from build123d import *

# Parameters (mm, degrees)
SKETCH1_W           = 85
SKETCH1_H           = 77
BOSS_EXTRUDE1_DEPTH = 1.75
SKETCH3_R           = 17.907
SKETCH3_R_2         = 13.97
BOSS_EXTRUDE3_DEPTH = 4.7625
BOSS_EXTRUDE7_DEPTH = 26
SKETCH6_W           = 77
SKETCH6_H           = 5
BOSS_EXTRUDE8_DEPTH = 2.5


with BuildPart() as part:
    # Sketch1 → Boss-Extrude1 (new body)
    with BuildSketch(Plane(origin=(0, 0, 0), x_dir=(1, 0, 0), z_dir=(0, 1, 0))):
        Rectangle(SKETCH1_W, SKETCH1_H)
    extrude(amount=BOSS_EXTRUDE1_DEPTH)

    # Sketch3 → Boss-Extrude3 (add)
    with BuildSketch(Plane(origin=(0, 1.75, 0), x_dir=(1, 0, 0), z_dir=(0, 1, 0))):
        with Locations((19.133331774, 19.92813227)):
            Circle(SKETCH3_R)
        with Locations((19.133331774, 19.92813227)):
            Circle(SKETCH3_R_2, mode=Mode.SUBTRACT)
        with Locations((-19.133331774, 19.92813227)):
            Circle(SKETCH3_R)
        with Locations((-19.133331774, 19.92813227)):
            Circle(SKETCH3_R_2, mode=Mode.SUBTRACT)
    extrude(amount=BOSS_EXTRUDE3_DEPTH)

    # Sketch4 → Boss-Extrude7 (add)
    with BuildSketch(Plane(origin=(0, 1.75, 0), x_dir=(1, 0, 0), z_dir=(0, 1, 0))):
        with BuildLine():
            ThreePointArc((-34.668002675, 28.83513227), (-31.887785522, 32.497323119), (-28.266663548, 35.330823584))
            Line((-28.266663548, 35.330823584), (-28.266663548, 37.83513227))
            Line((-28.266663548, 37.83513227), (-38.266663548, 37.83513227))
            Line((-38.266663548, 37.83513227), (-38.266663548, 28.83513227))
            Line((-38.266663548, 28.83513227), (-34.668002675, 28.83513227))
        make_face()
        with BuildLine():
            ThreePointArc((-28.266663548, 4.525440956), (-31.887785522, 7.358941421), (-34.668002675, 11.02113227))
            Line((-34.668002675, 11.02113227), (-38.266663548, 11.02113227))
            Line((-38.266663548, 11.02113227), (-38.266663548, 2.02113227))
            Line((-38.266663548, 2.02113227), (-28.266663548, 2.02113227))
            Line((-28.266663548, 2.02113227), (-28.266663548, 4.525440956))
        make_face()
        with BuildLine():
            Line((0, 11.02113227), (-3.598660873, 11.02113227))
            ThreePointArc((-3.598660873, 11.02113227), (-6.378878026, 7.358941421), (-10, 4.525440956))
            Line((-10, 4.525440956), (-10, 2.02113227))
            Line((-10, 2.02113227), (0, 2.02113227))
            Line((0, 2.02113227), (0, 11.02113227))
        make_face()
        with BuildLine():
            ThreePointArc((10, 4.525440956), (6.378878026, 7.358941421), (3.598660873, 11.02113227))
            Line((3.598660873, 11.02113227), (0, 11.02113227))
            Line((0, 11.02113227), (0, 2.02113227))
            Line((0, 2.02113227), (10, 2.02113227))
            Line((10, 2.02113227), (10, 4.525440956))
        make_face()
        with BuildLine():
            Line((0, 28.83513227), (0, 37.83513227))
            Line((0, 37.83513227), (-10, 37.83513227))
            Line((-10, 37.83513227), (-10, 35.330823584))
            ThreePointArc((-10, 35.330823584), (-6.378878026, 32.497323119), (-3.598660873, 28.83513227))
            Line((-3.598660873, 28.83513227), (0, 28.83513227))
        make_face()
        with BuildLine():
            Line((10, 37.83513227), (0, 37.83513227))
            Line((0, 37.83513227), (0, 28.83513227))
            Line((0, 28.83513227), (3.598660873, 28.83513227))
            ThreePointArc((3.598660873, 28.83513227), (6.378878026, 32.497323119), (10, 35.330823584))
            Line((10, 35.330823584), (10, 37.83513227))
        make_face()
        with BuildLine():
            Line((28.266663548, 37.83513227), (28.266663548, 35.330823584))
            ThreePointArc((28.266663548, 35.330823584), (31.887785522, 32.497323119), (34.668002675, 28.83513227))
            Line((34.668002675, 28.83513227), (38.266663548, 28.83513227))
            Line((38.266663548, 28.83513227), (38.266663548, 37.83513227))
            Line((38.266663548, 37.83513227), (28.266663548, 37.83513227))
        make_face()
        with BuildLine():
            ThreePointArc((34.668002675, 11.02113227), (31.887785522, 7.358941421), (28.266663548, 4.525440956))
            Line((28.266663548, 4.525440956), (28.266663548, 2.02113227))
            Line((28.266663548, 2.02113227), (38.266663548, 2.02113227))
            Line((38.266663548, 2.02113227), (38.266663548, 11.02113227))
            Line((38.266663548, 11.02113227), (34.668002675, 11.02113227))
        make_face()
    extrude(amount=BOSS_EXTRUDE7_DEPTH)

    # Sketch6 → Boss-Extrude8 (add)
    with BuildSketch(Plane.ZY.offset(42.5)):
        with Locations((0, -0.75)):
            Rectangle(SKETCH6_W, SKETCH6_H)
    boss_extrude8 = extrude(amount=BOSS_EXTRUDE8_DEPTH)

    # Mirror1: Boss-Extrude8 across plane
    add(boss_extrude8.mirror(Plane(origin=(0, 0, 0), x_dir=(0, 0, 1), z_dir=(1, 0, 0))))


solid = part.part
Geometry check sheet. Reference: the model listing, model coordinates, mm. A direction names the side the tool comes from. Round coordinates to 2 decimals unless told otherwise and drop trailing zeros. Order: outer loops, then holes, each group sorted by start corner. A loop starts at its lowest first (then second) coordinate and runs counter-clockwise, first axis right, second up. Notation, with made-up numbers: (-36, 39.5) -> (-15, 39.5) arc R35 cw to (-15, 74.5) -> close; hole circle Ø10 at (-29, 46.25). An arc over 180 degrees is marked (long way). Use one line per item in the form item = value.
1. Go/stop test with flat-tipped pins: pin 1 (6 mm diameter, centred on x = 1.5, z = -16, fed in from +Y); pin 2 (1 mm diameter, centred on x = 8, z = 23, fed in from -Y); pin 3 (3 mm diameter, centred on y = 16, z = -36.5, fed in from -X); pin 4 (2 mm diameter, centred on x = 34, z = -10.5, fed in from +Y). Record where each tip stops, or that it passes through.
Working result:
pin_1 = 6.51
pin_2 = 0
pin_3 = -38.27
pin_4 = 27.75
2. Set-up check for faces 4 (the face through (-38.267, 15, -7)), 5 (the face through (44, -3.25, -1)), 6 (the face through (31.842, 16.983, -32.543)): record each of +Z, -Z, +X, -X, +Y, -Y from which the full face is reachable in a straight line by a thin tool's end or side.
Working result:
face_4 = +Z, -Z, -X, +Y
face_5 = +Z, -Z, +X, -X, -Y
face_6 = +Y
3. Scan lines: line 1 along Z through (x, y) = (3, 22); line 2 along X through (y, z) = (-1.5, 11.5); line 3 along X through (y, z) = (24.5, -29). Record each from-to range of solid material in increasing order. Write a range as from..to.
Working result:
line_1 = -37.84..-28.84, -11.02..-2.02
line_2 = -45..-42.5, 42.5..45
line_3 = -38.27..-34.57, -3.69..3.69, 34.57..38.27
4. Cross-section at A-A, the plane y = 10.5. Count the separate pieces of the cut face and the enclosed holes in it, plus the area to 3 significant figures.
Working result:
separate_pieces = 6
enclosed_holes = 0
area = 525 mm^2
5. Mould release check, pull along X, two halves, no side actions. Record for faces 1 (the face through (38.267, 15, -6)), 2 (the face through (10, 15, -3)), 3 (the face through (-33, 15, -37.835)): pulls with the +X half, pulls with the -X half, needs draft (parallel to the pull), parting line crosses it, or undercut.
Working result:
face_1 = pulls with the +X half
face_2 = undercut
face_3 = needs draft
6. Cross-section at B-B, the plane z = 22. Enter the section's corners in (x, y), plus the area to 3 significant figures.
Working result:
outline = (-45, -3.25) -> (-42.5, -3.25) -> (-42.5, 0) -> (42.5, 0) -> (42.5, -3.25) -> (45, -3.25) -> (45, 1.75) -> (-45, 1.75) -> close
area = 174 mm^2
7. Cross-section at D-D, the plane x = 8. Enter the section's corners in (y, z), plus the area to 3 significant figures.
Working result:
outline = (0, -38.5) -> (1.75, -38.5) -> (1.75, -37.84) -> (27.75, -37.84) -> (27.75, -33.95) -> (6.51, -33.95) -> (6.51, -28.37) -> (1.75, -28.37) -> (1.75, -11.49) -> (6.51, -11.49) -> (6.51, -5.9) -> (27.75, -5.9) -> (27.75, -2.02) -> (1.75, -2.02) -> (1.75, 38.5) -> (0, 38.5) -> close
area = 390 mm^2
